Geometry: final body of the model. Coordinates: model frame, mm. Round coordinates to 2 decimals unless told otherwise and drop trailing zeros. Loops run counter-clockwise (first coordinate to the right, second up) from the corner with the lowest first, then second, coordinate; pieces in that order, holes last. Notation, with made-up numbers: M 3.5,44 L 8.5,44 A33 cw 8.5,72 Z; hole C 58,11.5 d8. An arc over 180 degrees is marked long. Write each question's results on one line, items separated by ' | '.
```python
from build123d import *

# Parameters (mm, degrees)
SKETCH1_W           = 25
SKETCH1_H           = 7
SKETCH1_R           = 1.75
BOSS_EXTRUDE1_DEPTH = 5
FILLET1_R           = 3
FILLET2_R           = 3


with BuildPart() as part:
    # Sketch1 → Boss-Extrude1 (new body)
    with BuildSketch(Plane.XY):
        Rectangle(SKETCH1_W, SKETCH1_H)
        with Locations((-9.635416667, 0)):
            Circle(SKETCH1_R, mode=Mode.SUBTRACT)
    extrude(amount=BOSS_EXTRUDE1_DEPTH)

    # Fillet1
    fillet1_edges = [part.edges().sort_by_distance(p)[0] for p in [
        (-12.5, -3.5, 2.5),
        (-12.5, 3.5, 2.5),
    ]]
    fillet(fillet1_edges, radius=FILLET1_R)

    # Fillet2
    fillet2_edges = [part.edges().sort_by_distance(p)[0] for p in [
        (12.5, -3.5, 2.5),
        (12.5, 3.5, 2.5),
    ]]
    fillet(fillet2_edges, radius=FILLET2_R)


solid = part.part
```
1. Section C-C (y = -1.25). Output: boundary loops of the cut face in (x, z), then the cut area to 3 significant figures.
Answer key:
outline: M -12.4,0 L -10.86,0 L -10.86,5 L -12.4,5 Z; M -8.41,0 L 12.4,0 L 12.4,5 L -8.41,5 Z | area: 112 mm²
2. Section B-B (y = 0). Output: boundary loops of the cut face in (x, z), then the cut area to 4 significant figures.
Answer key:
outline: M -12.5,0 L -11.39,0 L -11.39,5 L -12.5,5 Z; M -7.89,0 L 12.5,0 L 12.5,5 L -7.89,5 Z | area: 107.5 mm²
3. Draft query along Y for faces 1 (the face through (0, -3.5, 2)), 2 (the face through (0, 3.5, 2)), 3 (the face through (-11.384, 0.077, 2.465)). Return one class per face: pulls with the +Y half, pulls with the -Y half, needs draft (parallel to the pull), parting line crosses it, or undercut.
Answer key:
face 1: pulls with the -Y half | face 2: pulls with the +Y half | face 3: undercut
4. Section D-D (x = 10.5). Output: boundary loops of the cut face in (y, z).
Answer key:
outline: M -3.33,0 L 3.33,0 L 3.33,5 L -3.33,5 Z
5. Ray query, probe 1 along X at (y, z) = (-1.5, 4.45); probe 2 along X at (y, z) = (-1.25, 1.75); probe 3 along Y at (x, z) = (11.5, 3.65). Return the intervals inside material, ascending.
Answer key:
probe 1: x = -12.33 to -10.54, -8.73 to 12.33 | probe 2: x = -12.4 to -10.86, -8.41 to 12.4 | probe 3: y = -2.74 to 2.74
6. Pin query (flat end, axial travel): P1, Ø3, axis at y = 1, z = 3, coming from the -X side; P2, Ø3, axis at x = -9.64, y = 0, coming from the -Z side. Return the tip coordinate at first contact, or that it passes through.
Answer key:
P1: stops at x = -12.5 | P2: passes through
7. Section A-A (z = 0.8). Output: boundary loops of the cut face in (x, y), then the cut area to 3 significant figures.
Answer key:
outline: M -12.5,-0.5 A3 ccw -9.5,-3.5 L 9.5,-3.5 A3 ccw 12.5,-0.5 L 12.5,0.5 A3 ccw 9.5,3.5 L -9.5,3.5 A3 ccw -12.5,0.5 Z; hole C -9.64,0 d3.5 | area: 158 mm²
